Study the drawing (mm; zero at the part's minimum x, y, z) and answer. A direction names the side the tool comes from. Coordinates: 2 decimals unless noted, no trailing zeros. Loops run counter-clockwise (first coordinate to the right, second up) from the corner with the lowest first, then second, coordinate; pieces in that order, holes last. Notation, with made-up numbers: M -5,89.25 L 52,89.25 A34 ccw 52,124.25 Z; hole C 62,-33 d9. An arc over 180 degrees is marked long. Use one line per item in the form item = value. Start each with the question number.
1. The part is cut by section D-D (y = 20.25). Give the vertices of the cut face in (x, z).
2. The part is cut by section A-A (y = 5.5). Give the vertices of the cut face in (x, z), plus the area to 3 significant figures.
3. The part is cut by section C-C (x = 52). Give the vertices of the cut face in (y, z).
4. Find the intervals of material crossed by probe 1 along Z at (x, y) = (79.5, 4.75); probe 2 along X at (y, z) = (27, 54); probe 3 along X at (y, z) = (3.75, 34), in increasing order. Write a range as [from, to].
5. For a pull along X with two mould halves and no side action, classify the marked faces 1, 2 and 3 as released by +X, released by -X, zero draft, split by the parting line, or undercut.
6. Flat-ended cylindrical pins translate along their axes: pin 1 (20 mm diameter, centred on x = 69, z = 26.5, fed in from +Y); pin 2 (3.5 mm diameter, centred on y = 7, z = 24.5, fed in from -X); pin 3 (1.5 mm diameter, centred on y = 9.5, z = 93, fed in from -X); pin 4 (8 mm diameter, centred on x = 33.5, y = 6, fed in from +Z). Find the tip coordinate at first contact, or state that the pin passes through.
7. A tool of negligible diameter and unlimited length cuts with its end or side. For the marked faces 4 and 5, from which of +Z, -Z, +X, -X, +Y, -Y can it reach the whole face along a straight path? Write none if from no direction.
8. The part is cut by section B-B (z = 58.5). Give the vertices of the cut face in (x, y).
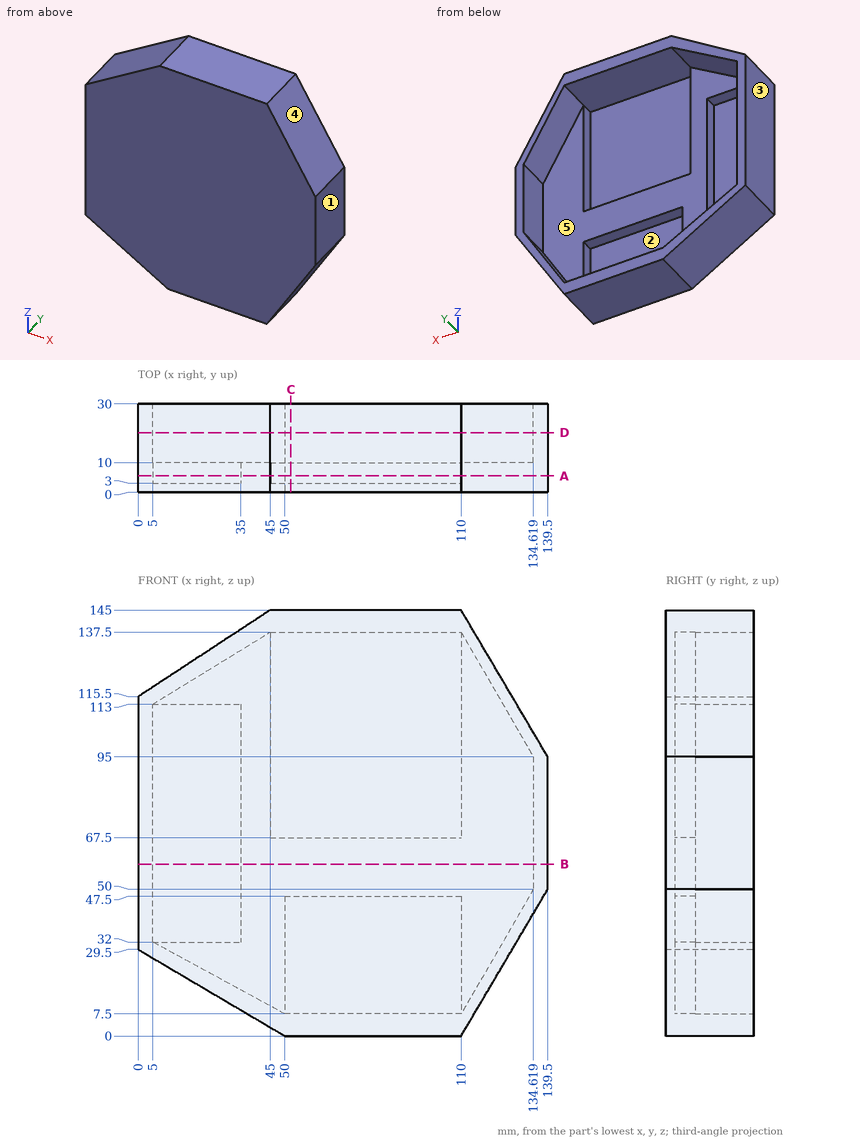
Computed values:
q1.outline = M 0,29.5 L 50,0 L 110,0 L 139.5,50 L 139.5,95 L 110,145 L 45,145 L 0,115.5 Z; hole M 5,32 L 50,7.5 L 110,7.5 L 134.62,50 L 134.62,95 L 110,137.5 L 45,137.5 L 5,113 Z
q2.outline = M 0,29.5 L 50,0 L 110,0 L 139.5,50 L 139.5,95 L 110,145 L 45,145 L 0,115.5 Z; hole M 5,32 L 35,32 L 35,113 L 5,113 Z; hole M 45,67.5 L 110,67.5 L 110,137.5 L 45,137.5 Z; hole M 50,7.5 L 110,7.5 L 110,47.5 L 50,47.5 Z
q2.area = 7,970 mm²
q3.outline = M 0,0 L 30,0 L 30,7.5 L 3,7.5 L 3,47.5 L 10,47.5 L 10,67.5 L 3,67.5 L 3,137.5 L 30,137.5 L 30,145 L 0,145 Z
q4.probe_1 = [0, 7.5], [47.5, 67.5], [137.5, 145]
q4.probe_2 = [0, 5], [134.62, 139.5]
q4.probe_3 = [0, 5], [35, 50], [110, 130.06]
q5.face_1 = released by +X
q5.face_2 = undercut
q5.face_3 = released by -X
q6.pin_1 = 3
q6.pin_2 = 5.51
q6.pin_3 = 0
q6.pin_4 = 140.08
q7.face_4 = +Z, +X, +Y, -Y
q7.face_5 = +Y
q8.outline = M 0,0 L 139.5,0 L 139.5,30 L 134.62,30 L 134.62,10 L 35,10 L 35,3 L 5,3 L 5,30 L 0,30 Z
